Read the model definition and answer for the solid it produces. Units are mm, in the model's axes. A direction names the side the tool comes from. Give positions to 0.01 mm unless a question says otherwise; leave off trailing zeros. Loops run counter-clockwise (first coordinate to the right, second up) from the corner with the lowest first, then second, coordinate; pieces in that order, holes last. Notation, with made-up numbers: (81.25, 37.25) -> (90.25, 37.25) arc R22 ccw to (90.25, 60.25) -> close; hole circle Ø7 at (82.25, 4.5). An arc over 180 degrees is marked (long way). One line per item, written item: value. Start each with the question number.
from build123d import *

# Parameters (mm, degrees)
SKETCH1_R           = 15
SKETCH1_R_2         = 11
BOSS_EXTRUDE1_DEPTH = 11.66


with BuildPart() as part:
    # Sketch1 → Boss-Extrude1 (new body)
    with BuildSketch(Plane(origin=(0, 0, 0), x_dir=(1, 0, 0), z_dir=(0, 1, 0))):
        Circle(SKETCH1_R)
        Circle(SKETCH1_R_2, mode=Mode.SUBTRACT)
    extrude(amount=BOSS_EXTRUDE1_DEPTH)

    # Sketch2 → Revolve1 (revolve)
    with BuildSketch(Plane.XY):
        Polygon((15, 11.66), (17, 11.66), (17, 10.66), (15, 10.33), align=None)
        Polygon((15, 0.33), (17, 0), (17, -1), (15, -1), (9, -1), (9, 0.33), (9, 4.66), (15, 4.66), align=None)
    revolve(axis=Axis((0, 0, 0), (0, 1, 0)))


solid = part.part
Item 1: For faces 4 (the cylindrical face through (-1.172, 1.79, -8.923)), 5 (the cylindrical face through (-2.38, 8.11, 10.74)), 6 (the cylindrical face through (-14.985, 5.26, -0.66)), determine the directions among +Z, -Z, +X, -X, +Y, -Y from which every point of the face is accessible in a straight line to the end or side of a thin tool.
Item 2: Flat-ended cylindrical pins translate along their axes: pin 1 (2 mm diameter, centred on y = 6, z = 0, fed in from -X); pin 2 (4 mm diameter, centred on x = -9, y = 1, fed in from +Z); pin 3 (11 mm diameter, centred on x = 4.5, z = -1.5, fed in from +Y). Find the tip coordinate at first contact, or state that the pin passes through.
Item 3: Section B-B, the plane z = 0 is taken. Determine the outline of the cut face in (x, y).
Item 4: Section A-A, the plane x = 0 is taken. Determine the outline of the cut face in (y, z), plus the area to 3 significant figures.
Item 5: Determine the mould class of faces 1 (the flat face through (-2, 4.66, 9)), 2 (the flat face through (-4, 11.66, 11)), 3 (the cylindrical face through (9.139, 11.153, -14.334)) for opening direction Z: pulls with the +Z half, pulls with the -Z half, needs draft (parallel to the pull), parting line crosses it, or undercut.
Item 6: Section C-C, the plane y = 8 is taken. Determine the outline of the cut face in (x, z).
Item 7: Consider L1, parallel to Z at x = 0, y = 2.3; L2, parallel to X at y = 9.25, z = 0. Determine where each line is inside the solid, lowest interval first. Write a range as [from, to].
Item 8: Section D-D, the plane y = 1 is taken. Determine the outline of the cut face in (x, z), plus the area to 3 significant figures.
Computed values:
1. face 4: +Y, -Y
1. face 5: +Y
1. face 6: none
2. pin 1: x = -15
2. pin 2: z = 15.37
2. pin 3: y = 4.66
3. outline: (-17, -1) -> (-9, -1) -> (-9, 4.66) -> (-11, 4.66) -> (-11, 11.66) -> (-17, 11.66) -> (-17, 10.66) -> (-15, 10.33) -> (-15, 0.33) -> (-17, 0) -> close; (9, -1) -> (17, -1) -> (17, 0) -> (15, 0.33) -> (15, 10.33) -> (17, 10.66) -> (17, 11.66) -> (11, 11.66) -> (11, 4.66) -> (9, 4.66) -> close
4. outline: (-1, -17) -> (0, -17) -> (0.33, -15) -> (10.33, -15) -> (10.66, -17) -> (11.66, -17) -> (11.66, -11) -> (4.66, -11) -> (4.66, -9) -> (-1, -9) -> close; (-1, 9) -> (4.66, 9) -> (4.66, 11) -> (11.66, 11) -> (11.66, 17) -> (10.66, 17) -> (10.33, 15) -> (0.33, 15) -> (0, 17) -> (-1, 17) -> close
4. area: 133 mm²
5. face 1: undercut
5. face 2: needs draft
5. face 3: parting line crosses it
6. outline: circle Ø30 at (0, 0); hole circle Ø22 at (0, 0)
7. L1: [-15, -9], [9, 15]
7. L2: [-15, -11], [11, 15]
8. outline: circle Ø30 at (0, 0); hole circle Ø18 at (0, 0)
8. area: 452 mm²
